Autodesk Inventor part; units mm, degrees
ref_plane "YZ Plane" through (0, 0, 0) normal (1, 0, 0) x (0, 1, 0)
ref_plane "XZ Plane" through (0, 0, 0) normal (0, 1, 0) x (-1, 0, 0)
ref_plane "XY Plane" through (0, 0, 0) normal (0, 0, 1) x (1, 0, 0)
sketch "Sketch1" plane through (0, 0, 0) normal (0, 1, 0) x (-1, 0, 0)
  line L0 (-26.4056, 15.9) -> (8.8944, 15.9)
  line L1 (8.8944, 15.9) -> (8.8944, -15.9)
  line L2 (8.8944, -15.9) -> (-26.4056, -15.9)
  line L3 (-26.4056, -15.9) -> (-26.4056, 15.9)
  line L4 (6.4944, 13.5) -> (-24.0056, 13.5)
  line L5 (-24.0056, 13.5) -> (-24.0056, -13.5)
  line L6 (-24.0056, -13.5) -> (6.4944, -13.5)
  line L7 (6.4944, -13.5) -> (6.4944, 13.5)
  point P0 (0, 0)
  dimension "d4" = 27
  dimension "d5" = 30.5
  dimension "d7" = 2.4
  dimension "d8" = 2.4
  dimension "d9" = 2.4
  dimension "d10" = 2.4
extrude "Extrusion1" add sketch "Sketch1" along normal blind 14
sketch "Sketch2" plane through (0, 0, 0) normal (0, -1, 0) x (1, 0, 0)
  circle A0 centre (8.7556, 18) radius 1.4
  circle A1 centre (8.7556, -18) radius 1.4
  line L0 (24.0056, -13.5) -> (24.0056, 13.5)
  circle A2 centre (8.7556, 18) radius 4.5
  circle A3 centre (8.7556, -18) radius 4.5
  line L1 (-6.4944, -13.5) -> (24.0056, -13.5)
  point P0 (0, 0)
  dimension "d13" = 36
  dimension "d14" = 15.25
  dimension "d15" = 2.8
  dimension "d16" = 18
extrude "Extrusion2" add sketch "Sketch2" against normal blind 10
fillet "Fillet1" radius 2 4 edges at (12.7355, 5, -15.9) (4.7756, 5, -15.9) (4.7756, 5, 15.9) (12.7355, 5, 15.9)
sketch "Sketch3" plane through (0, 0, 0) normal (0, -1, 0) x (1, 0, 0)
  circle A0 centre (8.7556, -18) radius 1.4
  circle A1 centre (8.7556, 18) radius 1.4
  line L0 (26.4056, -15.9) -> (15.2548, -15.9)
  line L1 (26.4056, 15.9) -> (26.4056, -15.9)
  line L2 (15.2548, 15.9) -> (26.4056, 15.9)
  arc A2 (13.255, 17.9308) -> (15.2548, 15.9) centre (15.2548, 17.9) ccw
  arc A3 (13.255, 17.9308) -> (4.2561, 17.9308) centre (8.7556, 18) ccw
  arc A4 (2.2563, 15.9) -> (4.2561, 17.9308) centre (2.2563, 17.9) ccw
  line L3 (-8.8944, 15.9) -> (2.2563, 15.9)
  line L4 (-8.8944, -15.9) -> (-8.8944, 15.9)
  line L5 (2.2563, -15.9) -> (-8.8944, -15.9)
  arc A5 (4.2561, -17.9308) -> (2.2563, -15.9) centre (2.2563, -17.9) ccw
  arc A6 (4.2561, -17.9308) -> (13.255, -17.9308) centre (8.7556, -18) ccw
  arc A7 (15.2548, -15.9) -> (13.255, -17.9308) centre (15.2548, -17.9) ccw
  line L6 (-6.4944, -13.5) -> (24.0056, -13.5)
  line L7 (-6.4944, 13.5) -> (-6.4944, -13.5)
  line L8 (24.0056, 13.5) -> (-6.4944, 13.5)
  line L9 (24.0056, -13.5) -> (24.0056, 13.5)
  line L10 (26.4056, 15.9) -> (26.4056, -15.9)
  line L11 (26.4056, -15.9) -> (-8.8944, -15.9)
  line L12 (-8.8944, -15.9) -> (-8.8944, -43)
  line L13 (-8.8944, -43) -> (26.4056, -43)
  line L14 (26.4056, -43) -> (26.4056, -15.9)
  circle A8 centre (18.7556, -38) radius 2.75
  circle A9 centre (-1.2444, -38) radius 2.75
  line L15 (-8.8944, -15.9) -> (-8.8944, 15.9)
  point P0 (0, 0)
  dimension "d20" = 5.5
  dimension "d21" = 20
  dimension "d22" = 20
  dimension "d23" = 5
  dimension "d25" = 10
extrude "Extrusion3" add sketch "Sketch3" against normal blind 4 contours L14 L13 L12 L5 A5 A6 A7 L0
fillet "Fillet2" radius 3 2 edges at (26.4056, 2, -43) (-8.8944, 2, -43)
sketch "Sketch4" plane through (0, 14, 0) normal (0, 1, 0) x (1, 0, 0)
  line L0 (-1.1926, 8) -> (-11.7963, 8)
  line L1 (-11.7963, 8) -> (-11.7963, -8)
  line L2 (-11.7963, -8) -> (-1.1926, -8)
  line L3 (-1.1926, -8) -> (-1.1926, 8)
  line L4 (-6.4944, -13.5) -> (-6.4944, 13.5)
  line L5 (-1.1926, 8) -> (-11.7963, -8) construction
  line L6 (-11.7963, 8) -> (-1.1926, -8) construction
  point P0 (0, 0)
  point P1 (-6.4944, 0)
  dimension "d29" = 8
extrude "Extrusion4" cut sketch "Sketch4" against normal through all
fillet "Fillet3" radius 1 2 edges at (-8.8944, 7, -8) (-8.8944, 7, 8)
properties part number "SocketMount"
Work out the finished part from the listing and answer in its coordinate system (mm). A direction names the side the tool comes from. Give positions to 0.01 mm unless a question says otherwise; leave off trailing zeros. Loops run counter-clockwise (first coordinate to the right, second up) from the corner with the lowest first, then second, coordinate; pieces in that order, holes last. Notation, with made-up numbers: (15.5, 6) -> (33.5, 6) arc R16 cw to (33.5, 18) -> close; hole circle Ø2 at (87.5, 25.5). An arc over 180 degrees is marked (long way). Write item = value, one per line. Start each with the question number.
(1) Given pin 1 Ø6.5 at (x, z) = (18.76, -38) entering from +Y; pin 2 Ø1 at (x, y) = (14, 2.5) entering from +Z; pin 3 Ø4 at (x, y) = (4, 7.5) entering from +Z, each flat-ended and moving along its own axis, determine where each tip first touches the part or whether it passes through.
(2) Which of the six approach directions +Z, -Z, +X, -X, +Y, -Y give full straight-line access (tool end or side, diameter ignored) to faces 5 (the flat face through (24.006, 7, 0)), 6 (the flat face through (9, 11, -15.9)), 7 (the flat face through (9, 10, 20)), 8 (the flat face through (-7, 7, -8))?
(3) Find section B-B on x = -1.5. Give the vertices of the cut face in (y, z), and give its area (3 significant figures).
(4) Find section C-C on z = -38. Give the vertices of the cut face in (x, y).
(5) Find section A-A on z = 11. Give the vertices of the cut face in (x, y), and give its area (3 significant figures).
(6) The mould has two halves that part along Z. Classify faces 1 (the cylindrical face through (-1.602, 1.972, -35.273)), 2 (the flat face through (9, 10, -20)), 3 (the flat face through (-7, 7, 8)), 4 (the flat face through (9, 2, -43)): +Z half, -Z half, draft (parallel to the pull), parting line (faces both ways), or undercut.
(7) Find section D-D on x = 12.5. Give the vertices of the cut face in (y, z).
(8) Find the intervals of material crossed by probe 1 along Z at (x, y) = (-6, 11.5); probe 2 along X at (y, z) = (9.25, -13); probe 3 along Z at (x, y) = (2.5, 1), in increasing order. Write a range as from..to.
From the geometry:
q1.pin_1 = 4
q1.pin_2 = 16.94
q1.pin_3 = 21.56
q2.face_5 = +Y, -Y
q2.face_6 = -Z, +Y
q2.face_7 = +Z, +X, -X, +Y
q2.face_8 = -X, +Y, -Y
q3.outline = (0, -43) -> (4, -43) -> (4, -40.74) -> (0, -40.74) -> close; (0, -35.26) -> (4, -35.26) -> (4, -15.9) -> (14, -15.9) -> (14, -13.5) -> (0, -13.5) -> close; (0, 13.5) -> (14, 13.5) -> (14, 15.9) -> (0, 15.9) -> close
q3.area = 154 mm^2
q4.outline = (-8.89, 0) -> (-3.99, 0) -> (-3.99, 4) -> (-8.89, 4) -> close; (1.51, 0) -> (16.01, 0) -> (16.01, 4) -> (1.51, 4) -> close; (21.51, 0) -> (26.41, 0) -> (26.41, 4) -> (21.51, 4) -> close
q5.outline = (-8.89, 0) -> (-6.49, 0) -> (-6.49, 14) -> (-8.89, 14) -> close; (24.01, 0) -> (26.41, 0) -> (26.41, 14) -> (24.01, 14) -> close
q5.area = 67.2 mm^2
q6.face_1 = undercut
q6.face_2 = draft
q6.face_3 = undercut
q6.face_4 = -Z half
q7.outline = (0, -43) -> (4, -43) -> (4, -20.5) -> (10, -20.5) -> (10, -15.9) -> (14, -15.9) -> (14, -13.5) -> (0, -13.5) -> close; (0, 13.5) -> (14, 13.5) -> (14, 15.9) -> (10, 15.9) -> (10, 20.5) -> (0, 20.5) -> close
q8.probe_1 = -15.9..-13.5, 13.5..15.9
q8.probe_2 = -8.89..-6.49, 24.01..26.41
q8.probe_3 = -43..-13.5, 13.5..15.91
